from build123d import *

# Parameters (mm, degrees)
BOSS_EXTRUDE1_DEPTH         = 6.35
F_1_4_CLEARANCE_HOLE1_D     = 6.5278
F_1_4_CLEARANCE_HOLE1_DEPTH = 6.35
CUT_EXTRUDE1_DEPTH          = 6.35
CUT_EXTRUDE2_START          = -6.35
CUT_EXTRUDE2_DEPTH          = 6.35


with BuildPart() as part:
    # Sketch1 → Boss-Extrude1 (new body)
    with BuildSketch(Plane(origin=(0, 0, 0), x_dir=(1, 0, 0), z_dir=(0, 1, 0))):
        with BuildLine():
            Line((-101.6, 50.8), (101.6, 50.8))
            Line((101.6, 50.8), (101.6, 7.9375))
            Line((101.6, 7.9375), (89.172371939, 7.9375))
            ThreePointArc((89.172371939, 7.9375), (87.957352042, 7.695817516), (86.927307909, 7.00756403))
            Line((86.927307909, 7.00756403), (82.164807909, 2.24506403))
            ThreePointArc((82.164807909, 2.24506403), (81.234871939, 0), (82.164807909, -2.24506403))
            Line((82.164807909, -2.24506403), (86.927307909, -7.00756403))
            ThreePointArc((86.927307909, -7.00756403), (87.957352042, -7.695817516), (89.172371939, -7.9375))
            Line((89.172371939, -7.9375), (101.6, -7.9375))
            Line((101.6, -7.9375), (101.6, -50.8))
            Line((101.6, -50.8), (-101.6, -50.8))
            Line((-101.6, -50.8), (-101.6, 50.8))
        make_face()
    extrude(amount=BOSS_EXTRUDE1_DEPTH)

    # 1/4 Clearance Hole1
    with Locations(Plane(origin=(0, 6.35, 0), x_dir=(-1, 0, 0), z_dir=(0, 1, 0))):
        with Locations((-88.9, 38.1), (-88.9, -38.1), (88.9, 19.05)):
            Hole(F_1_4_CLEARANCE_HOLE1_D / 2, depth=F_1_4_CLEARANCE_HOLE1_DEPTH)

    # Sketch4 → Cut-Extrude1 (cut)
    with BuildSketch(Plane(origin=(0, 6.35, 0), x_dir=(1, 0, 0), z_dir=(0, 1, 0))):
        with BuildLine():
            Line((88.9, 41.3639), (101.6, 41.3639))
            Line((101.6, 41.3639), (101.6, 34.8361))
            Line((101.6, 34.8361), (88.9, 34.8361))
            ThreePointArc((88.9, 34.8361), (85.6361, 38.1), (88.9, 41.3639))
        make_face()
    cut_extrude1 = extrude(amount=-CUT_EXTRUDE1_DEPTH, mode=Mode.SUBTRACT)

    # Mirror1: Cut-Extrude1 across plane
    add(cut_extrude1.mirror(Plane.XY), mode=Mode.SUBTRACT)

    # Sketch5 → Cut-Extrude2 (cut)
    with BuildSketch(Plane(origin=(0, 6.35, 0), x_dir=(1, 0, 0), z_dir=(0, 1, 0)).offset(CUT_EXTRUDE2_START)):
        with BuildLine():
            Line((-90.4875, -15.7861), (-87.3125, -15.7861))
            ThreePointArc((-87.3125, -15.7861), (-84.0486, -19.05), (-87.3125, -22.3139))
            Line((-87.3125, -22.3139), (-90.4875, -22.3139))
            ThreePointArc((-90.4875, -22.3139), (-93.7514, -19.05), (-90.4875, -15.7861))
        make_face()
    extrude(amount=CUT_EXTRUDE2_DEPTH, mode=Mode.SUBTRACT)


solid = part.part
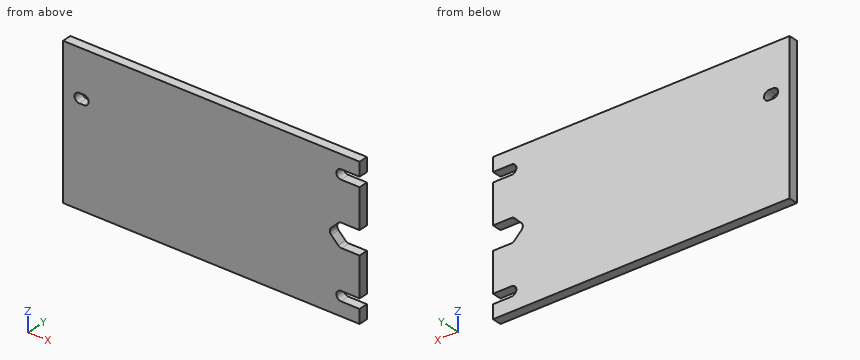
Work out the finished part from the listing and answer in its coordinate system (mm). Round coordinates to 2 decimals unless told otherwise and drop trailing zeros. Write each loop counter-clockwise with the first axis right and the second up, starting at its lowest first coordinate (ties: lowest second). Pieces come first, ordered by that corner, then holes. Notation, with made-up numbers: (89, 71.25) -> (127, 71.25) arc R21 cw to (127, 86.25) -> close; hole circle Ø8 at (17.25, 56.5). An arc over 180 degrees is marked (long way). Answer as CSV lines item,"result". Start each with the question number.
(1) The part is cut by section C-C, the plane z = -38.1. Give the vertices of the cut face in (x, y), then the cut area to 3 significant figures.
(2) The part is cut by section A-A, the plane z = 19.05. Give the vertices of the cut face in (x, y), then the cut area to 3 significant figures.
(3) Find the intervals of material crossed by probe 1 along X at (y, z) = (4.5, 20.5); probe 2 along X at (y, z) = (1, 40); probe 3 along Z at (x, y) = (-92, 2), in increasing order.
Output values:
1,outline,"(-101.6, 0) -> (85.64, 0) -> (85.64, 6.35) -> (-101.6, 6.35) -> close"
1,area,"1,190 mm²"
2,outline,"(-101.6, 0) -> (-93.75, 0) -> (-93.75, 6.35) -> (-101.6, 6.35) -> close; (-84.05, 0) -> (101.6, 0) -> (101.6, 6.35) -> (-84.05, 6.35) -> close"
2,area,"1,230 mm²"
3,probe 1,"x = -101.6 to -93.41, -84.39 to 101.6"
3,probe 2,"x = -101.6 to 86.25"
3,probe 3,"z = -50.8 to 16.16, 21.94 to 50.8"
